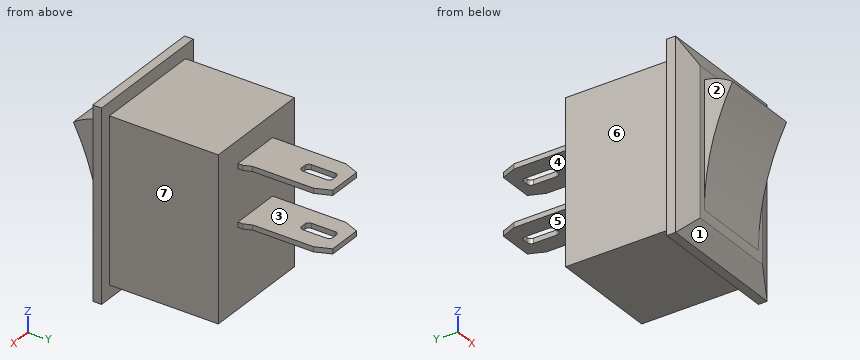
Autodesk Inventor part; units mm, degrees
ref_plane "作業平面1" through (0, 0, 4.5) normal (0, 0, 1) x (1, 0, 0)
ref_plane "YZ Plane" through (0, 0, 0) normal (1, 0, 0) x (0, 1, 0)
ref_plane "XZ Plane" through (0, 0, 0) normal (0, 1, 0) x (-1, 0, 0)
sketch "スケッチ1" plane through (0, 0, 0) normal (0, 1, 0) x (-1, 0, 0)
  line L0 (4.4, -6.5) -> (-4.4, -6.5)
  line L1 (-4.4, -6.5) -> (-4.4, 6.5)
  line L2 (-4.4, 6.5) -> (4.4, 6.5)
  line L3 (4.4, 6.5) -> (4.4, -6.5)
  line L4 (-4.4, 0) -> (0, 0) construction
  line L5 (0, 0) -> (0, -6.5) construction
  dimension "d0" = 13
  dimension "d1" = 8.8
extrude "押し出し1" add sketch "スケッチ1" along normal blind 8.7
sketch "スケッチ2" plane through (0, 0, 0) normal (0, -1, 0) x (1, 0, 0)
  line L0 (5.3, 7.55) -> (-5.3, 7.55)
  line L1 (-5.3, 7.55) -> (-5.3, -7.55)
  line L2 (-5.3, -7.55) -> (5.3, -7.55)
  line L3 (5.3, -7.55) -> (5.3, 7.55)
  line L4 (5.3, 0) -> (0, 0) construction
  line L5 (0, 0) -> (0, -7.55) construction
  dimension "d4" = 15.1
  dimension "d5" = 10.6
extrude "押し出し2" add sketch "スケッチ2" along normal blind 1.5
sketch "スケッチ3" plane through (0, 0, 0) normal (0, 0, 1) x (1, 0, 0)
  line L0 (5.3, -1.5) -> (-5.3, -1.5) construction
  line L1 (-5.3, -1.5) -> (-5.3, -0.7)
  line L2 (-5.3, 0) -> (-5.3, -1.5) construction
  line L3 (-5.3, -0.7) -> (-3.6, -1.5)
  line L4 (-3.6, -1.5) -> (-5.3, -1.5)
  point P0 (0, 0)
  dimension "d8" = 1.7
  dimension "d9" = 0.8
sketch "スケッチ4" plane through (0, -1.5, 0) normal (0, -1, 0) x (1, 0, 0)
  line L0 (5.3, 7.55) -> (-5.3, 7.55) construction
  line L1 (-5.3, 7.55) -> (-5.3, -7.55) construction
  line L2 (-5.3, -7.55) -> (5.3, -7.55) construction
  line L3 (5.3, -7.55) -> (5.3, 7.55) construction
  line L4 (-3.6, 5.85) -> (3.6, 5.85)
  line L5 (3.6, 5.85) -> (3.6, -5.85)
  line L6 (3.6, -5.85) -> (-3.6, -5.85)
  line L7 (-3.6, -5.85) -> (-3.6, 5.85)
  point P0 (0, 0)
  dimension "d10" = 1.7
sweep "スイープ1" cut profiles "スケッチ3" path "スケッチ4"
sketch "スケッチ5" plane through (0, 0, 0) normal (1, 0, 0) x (0, 1, 0)
  line L0 (-1.5, 5.85) -> (-1.5, -5.85) construction
  arc A0 (-1.5, -5) -> (-3.75, 4.0973) centre (-21.0161, -5) ccw
  line L1 (-1.5, 5) -> (-1.5, -5)
  line L2 (-21.0161, -5) -> (-1.5, -5) construction
  arc A1 (-1.5, 5) -> (-3.75, 4.0973) centre (-0.8, 0) ccw
  line L3 (-0.8, 0) -> (0, 0) construction
  dimension "d16" = 2.25
  dimension "d17" = 0.8
  dimension "d18" = 10
extrude "押し出し3" add sketch "スケッチ5" along normal mid plane 6.25
sketch "スケッチ6" plane through (0, 0, 0) normal (0, 0, 1) x (1, 0, 0)
  line L0 (4.4, 8.7) -> (-4.4, 8.7) construction
  line L1 (0, 8.7) -> (0, 12.8003) construction
  line L2 (-1.875, 8.7) -> (-1.875, 14.55)
  line L3 (-1.875, 14.55) -> (-1.375, 15.75)
  line L4 (-1.375, 15.75) -> (1.375, 15.75)
  line L5 (1.375, 15.75) -> (1.875, 14.55)
  line L6 (1.875, 14.55) -> (1.875, 9.7)
  line L7 (1.875, 9.7) -> (2.125, 9.1)
  line L8 (2.125, 9.1) -> (2.125, 8.7)
  line L9 (2.125, 8.7) -> (-1.875, 8.7)
  line L10 (1.875, 14.55) -> (-1.875, 14.55) construction
  line L11 (0.2, 14.95) -> (-0.2, 14.95)
  line L12 (-0.5, 14.65) -> (-0.5, 12.75)
  line L13 (-0.2, 12.45) -> (0.2, 12.45)
  line L14 (0.5, 12.75) -> (0.5, 14.65)
  arc A0 (0.5, 14.65) -> (0.2, 14.95) centre (0.2, 14.65) ccw
  arc A1 (-0.2, 14.95) -> (-0.5, 14.65) centre (-0.2, 14.65) ccw
  arc A2 (-0.5, 12.75) -> (-0.2, 12.45) centre (-0.2, 12.75) ccw
  arc A3 (0.2, 12.45) -> (0.5, 12.75) centre (0.2, 12.75) ccw
  point P0 (0, 0)
  dimension "d21" = 3.75
  dimension "d22" = 2.75
  dimension "d23" = 1.2
  dimension "d24" = 7.05
  dimension "d25" = 0.25
  dimension "d26" = 0.4
  dimension "d27" = 0.3
  dimension "d28" = 2.5
  dimension "d29" = 1
  dimension "d30" = 0.8
extrude "押し出し4" add sketch "スケッチ6" along normal mid plane 0.4
ref_plane "作業平面1" through (0, 0, 4.5) normal (0, 0, 1) x (1, 0, 0)
sketch "スケッチ7" plane through (0, 0, 4.5) normal (0, 0, 1) x (1, 0, 0)
  arc A0 (0.5, 14.65) -> (0.2, 14.95) centre (0.2, 14.65) ccw
  line L0 (0.2, 14.95) -> (-0.2, 14.95)
  arc A1 (-0.2, 14.95) -> (-0.5, 14.65) centre (-0.2, 14.65) ccw
  line L1 (-0.5, 14.65) -> (-0.5, 12.75)
  arc A2 (-0.5, 12.75) -> (-0.2, 12.45) centre (-0.2, 12.75) ccw
  line L2 (-0.2, 12.45) -> (0.2, 12.45)
  arc A3 (0.2, 12.45) -> (0.5, 12.75) centre (0.2, 12.75) ccw
  line L3 (0.5, 12.75) -> (0.5, 14.65)
  line L4 (-1.875, 8.7) -> (-1.875, 14.55)
  line L5 (-1.875, 14.55) -> (-1.375, 15.75)
  line L6 (-1.375, 15.75) -> (1.375, 15.75)
  line L7 (1.375, 15.75) -> (1.875, 14.55)
  line L8 (1.875, 14.55) -> (1.875, 9.7)
  line L9 (1.875, 9.7) -> (2.125, 9.1)
  line L10 (2.125, 9.1) -> (2.125, 8.7)
  line L11 (-1.875, 8.7) -> (2.125, 8.7)
  point P0 (0, 0)
extrude "押し出し5" add sketch "スケッチ7" along normal mid plane 0.4
properties part number "switch_6A"
CAD build for the part. Positions are in the model's coordinates, mm. Face numbers are marked on the shaded views. A direction names the side the tool comes from. Round coordinates to 2 decimals unless told otherwise and drop trailing zeros. Loops run counter-clockwise (first coordinate to the right, second up) from the corner with the lowest first, then second, coordinate; pieces in that order, holes last. Notation, with made-up numbers: (-31, -38) - (-25, -38) arc R14 ccw to (-25, -19) - close; hole circle Ø4 at (61.25, 28). An arc over 180 degrees is marked (long way). Put each result on its own line as item: value.
1. Two-plate mould, pull along Z, no slides. Class the marked faces 1, 2 and 3: released by +Z, released by -Z, zero draft, split by the parting line, or undercut.
Geometry check:
face 1: released by -Z
face 2: zero draft
face 3: undercut
2. Wall check: line 1 (Z direction, x = -1, y = 11.25); line 2 (Y direction, x = 2, z = -4.75); line 3 (X direction, y = 2.5, z = 2). Give the ranges that are in metal, low to high.
Geometry check:
line 1: -0.2 to 0.2, 4.3 to 4.7
line 2: -1.5 to 8.7
line 3: -4.4 to 4.4
3. Pin check, flat tips, straight feed: P1, Ø1.8, axis at y = -2.5, z = -1, coming from the -X side (3 decimals); P2, Ø5, axis at y = 13, z = -4.5, coming from the +X side; P3, Ø5, axis at x = -4, z = -2, coming from the +Y side; P4, Ø2.5, axis at x = -1, y = 4, coming from the +Z side. Stop position of each tip, or through.
Geometry check:
P1: x = -3.125
P2: through
P3: y = 8.7
P4: z = 6.5
4. Slice it at B-B on y = 10.5. List the corners of the cut face in (x, z) (3 decimals).
Geometry check:
outline: (-1.875, -0.2) - (1.875, -0.2) - (1.875, 0.2) - (-1.875, 0.2) - close; (-1.875, 4.3) - (1.875, 4.3) - (1.875, 4.7) - (-1.875, 4.7) - close
5. Slice it at A-A on y = 13.25. List the corners of the cut face in (x, z) (3 decimals).
Geometry check:
outline: (-1.875, -0.2) - (-0.5, -0.2) - (-0.5, 0.2) - (-1.875, 0.2) - close; (-1.875, 4.3) - (-0.5, 4.3) - (-0.5, 4.7) - (-1.875, 4.7) - close; (0.5, -0.2) - (1.875, -0.2) - (1.875, 0.2) - (0.5, 0.2) - close; (0.5, 4.3) - (1.875, 4.3) - (1.875, 4.7) - (0.5, 4.7) - close
6. Slice it at C-C on z = -5.25. List the corners of the cut face in (x, y), and give its area (3 significant figures).
Geometry check:
outline: (-5.3, -0.7) - (-3.6, -1.5) - (3.6, -1.5) - (5.3, -0.7) - (5.3, 0) - (4.4, 0) - (4.4, 8.7) - (-4.4, 8.7) - (-4.4, 0) - (-5.3, 0) - close
area: 91.1 mm²
7. Slice it at D-D on x = 1. List the corners of the cut face in (y, z), and give its area (3 significant figures).
Geometry check:
outline: (-3.75, 4.1) arc R19.52 cw to (-1.5, -5) - (-1.5, -5.85) - (-0.7, -7.55) - (0, -7.55) - (0, -6.5) - (8.7, -6.5) - (8.7, -0.2) - (15.75, -0.2) - (15.75, 0.2) - (8.7, 0.2) - (8.7, 4.3) - (15.75, 4.3) - (15.75, 4.7) - (8.7, 4.7) - (8.7, 6.5) - (0, 6.5) - (0, 7.55) - (-0.7, 7.55) - (-1.5, 5.85) - (-1.5, 5) arc R5.05 ccw to start
area: 148 mm²
8. 3-axis set-ups, long thin cutter, end or side, ignore diameter. For the marked faces 4, 5, 6 and 7: which of +Z, -Z, +X, -X, +Y, -Y reach the whole face in a straight line?
Geometry check:
face 4: +X, -X, +Y
face 5: -Z, +X, -X, +Y
face 6: +Z, -Z, -X, +Y
face 7: +Z, -Z, +X, +Y
